```python
from build123d import *

# Parameters (mm, degrees)
SKETCH1_W           = 77
SKETCH1_H           = 14
BOSS_EXTRUDE1_DEPTH = 2
SKETCH3_W           = 9
SKETCH3_H           = 2
BOSS_EXTRUDE2_DEPTH = 10.5
SKETCH4_W           = 9
SKETCH4_H           = 2
BOSS_EXTRUDE3_DEPTH = 10.5
SKETCH5_W           = 10.5
SKETCH5_H           = 9
BOSS_EXTRUDE4_DEPTH = 6.5
SKETCH6_W           = 6.5
SKETCH6_H           = 2.5
CUT_EXTRUDE1_DEPTH  = 9
SKETCH8_R           = 1.5
CUT_EXTRUDE2_DEPTH  = 8.5
SKETCH10_W          = 9
SKETCH10_H          = 6
CUT_EXTRUDE4_DEPTH  = 2
CHAMFER1_SIZE       = 9
CHAMFER1_SIZE2      = 2
BOSS_EXTRUDE5_DEPTH = 5
SKETCH13_R          = 4
CUT_EXTRUDE5_DEPTH  = 5
FILLET3_R           = 1


with BuildPart() as part:
    # Sketch1 → Boss-Extrude1 (new body)
    with BuildSketch(Plane(origin=(0, 0, 0), x_dir=(1, 0, 0), z_dir=(0, 1, 0))):
        with Locations((-53.253755964, -5.729579977)):
            Rectangle(SKETCH1_W, SKETCH1_H)
    extrude(amount=BOSS_EXTRUDE1_DEPTH)

    # Sketch3 → Boss-Extrude2 (add)
    with BuildSketch(Plane.ZY.offset(91.753755964)):
        with Locations((5.729579977, 1)):
            Rectangle(SKETCH3_W, SKETCH3_H)
    extrude(amount=BOSS_EXTRUDE2_DEPTH)

    # Sketch4 → Boss-Extrude3 (add)
    with BuildSketch(Plane(origin=(-14.753755964, 0, 0), x_dir=(0, 0, -1), z_dir=(1, 0, 0))):
        with Locations((-5.729579977, 1)):
            Rectangle(SKETCH4_W, SKETCH4_H)
    extrude(amount=BOSS_EXTRUDE3_DEPTH)

    # Sketch5 → Boss-Extrude4 (add)
    with BuildSketch(Plane(origin=(0, 2, 0), x_dir=(1, 0, 0), z_dir=(0, 1, 0))):
        with Locations((-97.003755964, -5.729579977)):
            Rectangle(SKETCH5_W, SKETCH5_H)
        with Locations((-9.503755964, -5.729579977)):
            Rectangle(SKETCH5_W, SKETCH5_H)
    extrude(amount=BOSS_EXTRUDE4_DEPTH)

    # Sketch6 → Cut-Extrude1 (cut)
    with BuildSketch(Plane.XY.offset(10.229579977)):
        with Locations((-9.503755964, 5.25)):
            Rectangle(SKETCH6_W, SKETCH6_H)
        with Locations((-97.003755964, 5.25)):
            Rectangle(SKETCH6_W, SKETCH6_H)
    extrude(amount=-CUT_EXTRUDE1_DEPTH, mode=Mode.SUBTRACT)

    # Sketch8 → Cut-Extrude2 (cut)
    with BuildSketch(Plane(origin=(0, 8.5, 0), x_dir=(1, 0, 0), z_dir=(0, 1, 0))):
        with Locations((-88.178755964, -9.379579977)):
            Circle(SKETCH8_R)
        with Locations((-18.328755964, -9.379579977)):
            Circle(SKETCH8_R)
        with Locations((-97.003755964, -5.729579977)):
            Circle(SKETCH8_R)
        with Locations((-9.503755964, -5.729579977)):
            Circle(SKETCH8_R)
    extrude(amount=-CUT_EXTRUDE2_DEPTH, mode=Mode.SUBTRACT)

    # Sketch10 → Cut-Extrude4 (cut)
    with BuildSketch(Plane(origin=(0, 0, 0), x_dir=(-1, 0, 0), z_dir=(0, -1, 0))):
        with Locations((97.753755964, -5.729579977)):
            Rectangle(SKETCH10_W, SKETCH10_H)
        with Locations((8.753755964, -5.729579977)):
            Rectangle(SKETCH10_W, SKETCH10_H)
    extrude(amount=-CUT_EXTRUDE4_DEPTH, mode=Mode.SUBTRACT)

    # Chamfer1
    chamfer1_edges = [part.edges().sort_by_distance(p)[0] for p in [
        (-102.253755964, 0, 1.979579977),
        (-4.253755964, 0, 9.479579977),
        (-4.253755964, 0, 1.979579977),
        (-102.253755964, 0, 9.479579977),
    ]]
    chamfer1_side = [part.faces().sort_by_distance(p)[0] for p in [
        (-53.253755964, 0, 5.684508499),
    ]]
    chamfer(chamfer1_edges, length=CHAMFER1_SIZE, length2=CHAMFER1_SIZE2, reference=chamfer1_side[0])

    # Sketch12 → Boss-Extrude5 (add)
    with BuildSketch(Plane(origin=(0, 2, 0), x_dir=(1, 0, 0), z_dir=(0, 1, 0))):
        with BuildLine():
            Line((-26.753755964, -12.729579977), (-14.753755964, -12.729579977))
            Line((-14.753755964, -12.729579977), (-14.753755964, -18.729579977))
            ThreePointArc((-14.753755964, -18.729579977), (-20.753755964, -24.729579977), (-26.753755964, -18.729579977))
            Line((-26.753755964, -18.729579977), (-26.753755964, -12.729579977))
        make_face()
        with BuildLine():
            Line((-91.753755964, -12.729579977), (-91.753755964, -18.729579977))
            ThreePointArc((-91.753755964, -18.729579977), (-85.753755964, -24.729579977), (-79.753755964, -18.729579977))
            Line((-79.753755964, -18.729579977), (-79.753755964, -12.729579977))
            Line((-79.753755964, -12.729579977), (-91.753755964, -12.729579977))
        make_face()
    extrude(amount=-BOSS_EXTRUDE5_DEPTH)

    # Sketch13 → Cut-Extrude5 (cut)
    with BuildSketch(Plane(origin=(0, 2, 0), x_dir=(1, 0, 0), z_dir=(0, 1, 0))):
        with Locations((-85.753755964, -18.729579977)):
            Circle(SKETCH13_R)
        with Locations((-20.753755964, -18.729579977)):
            Circle(SKETCH13_R)
    extrude(amount=-CUT_EXTRUDE5_DEPTH, mode=Mode.SUBTRACT)

    # Fillet3
    fillet3_edges = [part.edges().sort_by_distance(p)[0] for p in [
        (-85.753755964, -3, 12.729579977),
        (-85.753755964, 2, 24.729579977),
        (-79.753755964, 2, 15.729579977),
        (-20.753755964, -3, 12.729579977),
        (-20.753755964, 2, 24.729579977),
        (-26.753755964, 2, 15.729579977),
        (-91.753755964, 8.5, 5.729579977),
        (-102.253755964, 8.5, 5.729579977),
        (-14.753755964, 8.5, 5.729579977),
        (-4.253755964, 8.5, 5.729579977),
        (-91.753755964, 1, -1.270420023),
        (-14.753755964, 1, -1.270420023),
    ]]
    fillet(fillet3_edges, radius=FILLET3_R)


solid = part.part
```
Geometry check sheet. Reference: the model listing, model coordinates, mm. A direction names the side the tool comes from. Give positions to 0.01 mm unless a question says otherwise; leave off trailing zeros. Loops run counter-clockwise (first coordinate to the right, second up) from the corner with the lowest first, then second, coordinate; pieces in that order, holes last. Notation, with made-up numbers: M -36.5,17.25 L 2.5,17.25 A17 ccw 2.5,28.25 Z; hole C 29,18.25 d2. An arc over 180 degrees is marked long. Answer as CSV lines item,"result".
Item 1: Access from +Z, -Z, +X, -X, +Y, -Y to the whole of each face (thin tool, end or side, straight path). Record for faces 1 (the flat face through (-91.754, 5, 6)), 2 (the flat face through (-86, -1, 12.73)), 3 (the flat face through (-7.7, 2, 5.7)).
Values:
face 1,"+Z, -Z, +Y"
face 2,"-Z, +X, -X, -Y"
face 3,"+X, -Y"
Item 2: Cross-section at D-D on z = 21.5. Count the separate pieces of the cut face and the enclosed holes in it, and give its area (3 significant figures).
Values:
separate pieces,"4"
enclosed holes,"0"
area,"47.8 mm²"
Item 3: Material ranges on line 1 (Z direction, x = -8, y = 1.5); line 2 (X direction, y = 2.75, z = 7.5); line 3 (X direction, y = 1.5, z = 20), recorded low to high.
Values:
line 1,"z = 1.23 to 2.73, 8.73 to 10.23"
line 2,"x = -102.25 to -91.75, -14.75 to -4.25"
line 3,"x = -91.48 to -89.55, -81.96 to -80.03, -26.48 to -24.55, -16.96 to -15.03"
Item 4: Cross-section at A-A on y = -1. Record the cut outline in (x, z).
Values:
outline,"M -91.75,12.73 L -79.75,12.73 L -79.75,18.73 A6 ccw -91.75,18.73 Z; M -26.75,12.73 L -14.75,12.73 L -14.75,18.73 A6 ccw -26.75,18.73 Z; hole C -85.75,18.73 d8; hole C -20.75,18.73 d8"
Item 5: Release check for a two-part mould opening along X. For faces 4 (the flat face through (-10, 3, 10.23)), 5 (the flat face through (-4.254, 5, 6)), 6 (the flat face through (-93.754, 5, 6)), 7 (the flat face through (-26.754, -1, 16)) record: pulls with the +X half, pulls with the -X half, needs draft (parallel to the pull), parting line crosses it, or undercut.
Values:
face 4,"needs draft"
face 5,"pulls with the +X half"
face 6,"undercut"
face 7,"undercut"
Item 6: Cross-section at C-C on y = 3. Record the cut outline in (x, z).
Values:
outline,"M -102.25,1.23 L -91.75,1.23 L -91.75,10.23 L -102.25,10.23 Z; M -14.75,1.23 L -4.25,1.23 L -4.25,10.23 L -14.75,10.23 Z; hole C -97,5.73 d3; hole C -9.5,5.73 d3"
Item 7: Cross-section at B-B on x = -76.5. Record the cut outline in (y, z), and give its area (3 significant figures).
Values:
outline,"M 0,-1.27 L 2,-1.27 L 2,12.73 L 0,12.73 Z"
area,"28.0 mm²"
Item 8: Depth check by flat-ended pin: P1, Ø0.6, axis at x = -23.5, y = -1, coming from the -Z side; P2, Ø12, axis at x = -62, z = 13.5, coming from the +Y side; P3, Ø5, axis at x = -91.5, y = 2.5, coming from the -Z side; P4, Ø4, axis at x = -9.5, z = 5.73, coming from the -Y side. Enter the tip coordinate at first touch or a pass-through.
Values:
P1,"stops at z = 12.73"
P2,"stops at y = 2"
P3,"stops at z = -1.27"
P4,"stops at y = 2"
